Part model, mm, in its own coordinate system. A direction names the side the tool comes from. Give positions to 0.01 mm unless a question says otherwise; leave off trailing zeros. Order: outer loops, then holes, each group sorted by start corner. A loop starts at its lowest first (then second) coordinate and runs counter-clockwise, first axis right, second up. Notation, with made-up numbers: M -29.75,56.5 L 4.25,56.5 A22 cw 4.25,74.5 Z; hole C -37,56 d7. An arc over 180 degrees is marked long. Answer as a JSON object with one key per item and string values.
from build123d import *

# Parameters (mm, degrees)
BOSS_EXTRUDE1_DEPTH = 20
CUT_EXTRUDE3_DEPTH  = 8
SKETCH4_W           = 7
SKETCH4_H           = 15
SKETCH4_R           = 2
BOSS_EXTRUDE2_DEPTH = 5


with BuildPart() as part:
    # Sketch1 → Boss-Extrude1 (new body)
    with BuildSketch(Plane(origin=(0, 0, 0), x_dir=(1, 0, 0), z_dir=(0, 1, 0))):
        Polygon((-1.5, -12.5), (-1.5, 4.5), (1.5, 4.5), (1.5, -12.5), (3.5, -12.5), (3.5, 12.5), (-3.5, 12.5), (-3.5, -12.5), align=None)
    extrude(amount=BOSS_EXTRUDE1_DEPTH)

    # Sketch2 → Cut-Extrude3 (cut)
    with BuildSketch(Plane.XY.offset(-4.5)):
        with BuildLine():
            Line((2, 17.5), (2, 10.5))
            ThreePointArc((2, 10.5), (0, 8.5), (-2, 10.5))
            Line((-2, 10.5), (-2, 17.5))
            ThreePointArc((-2, 17.5), (0, 19.5), (2, 17.5))
        make_face()
    extrude(amount=-CUT_EXTRUDE3_DEPTH, mode=Mode.SUBTRACT)

    # Sketch4 → Boss-Extrude2 (add)
    with BuildSketch(Plane(origin=(0, 0, -12.5), x_dir=(-1, 0, 0), z_dir=(0, 0, -1))):
        with Locations((0, -7.5)):
            Rectangle(SKETCH4_W, SKETCH4_H)
        with Locations((0, -4)):
            Circle(SKETCH4_R, mode=Mode.SUBTRACT)
        with Locations((0, -11)):
            Circle(SKETCH4_R, mode=Mode.SUBTRACT)
    extrude(amount=-BOSS_EXTRUDE2_DEPTH)


solid = part.part
1. Cut at A-A on y = -4. Give the cut face in (x, z).
Worked answers:
{"outline": "M -3.5,-12.5 L -2,-12.5 L -2,-7.5 L -3.5,-7.5 Z; M 2,-12.5 L 3.5,-12.5 L 3.5,-7.5 L 2,-7.5 Z"}
2. Cut at D-D on x = 0.5. Give the cut face in (y, z), plus the area to 3 significant figures.
Worked answers:
{"outline": "M -15,-12.5 L -12.94,-12.5 L -12.94,-7.5 L -15,-7.5 Z; M -9.06,-12.5 L -5.94,-12.5 L -5.94,-7.5 L -9.06,-7.5 Z; M -2.06,-12.5 L 8.56,-12.5 L 8.56,-4.5 L 0,-4.5 L 0,-7.5 L -2.06,-7.5 Z; M 19.44,-12.5 L 20,-12.5 L 20,-4.5 L 19.44,-4.5 Z", "area": "109 mm^2"}
3. Cut at B-B on z = -2.25. Give the cut face in (x, y), plus the area to 3 significant figures.
Worked answers:
{"outline": "M -3.5,0 L -1.5,0 L -1.5,20 L -3.5,20 Z; M 1.5,0 L 3.5,0 L 3.5,20 L 1.5,20 Z", "area": "80.0 mm^2"}
4. Cut at C-C on y = 2.5. Give the cut face in (x, z).
Worked answers:
{"outline": "M -3.5,-12.5 L 3.5,-12.5 L 3.5,12.5 L 1.5,12.5 L 1.5,-4.5 L -1.5,-4.5 L -1.5,12.5 L -3.5,12.5 Z"}
5. Pin check, flat tips, straight feed: P1, Ø4, axis at x = -2.5, z = 9.5, coming from the -Y side; P2, Ø3.5, axis at x = -0.5, y = -4.5, coming from the +Z side. Stop position of each tip, or through.
Worked answers:
{"P1": "stops at y = 0", "P2": "stops at z = -7.5"}
6. Two-plate mould, pull along X, no slides. Class faces 6 (the cylindrical face through (0, 19.5, -8.4)), 7 (the flat face through (2, 20, 0)), 8 (the flat face through (3.5, 6, -3)): +X half, -X half, draft (parallel to the pull), parting line (faces both ways), or undercut.
Worked answers:
{"face 6": "undercut", "face 7": "draft", "face 8": "+X half"}
7. Which spindle directions (+Z, -Z, +X, -X, +Y, -Y) get a long thin tool onto all of the face, cutting with end or side? Do faces 1 (the flat face through (0, -7, -7.5)), 2 (the flat face through (0, 19.7, -4.5)), 3 (the cylindrical face through (0, 8.5, -8.4)), 4 (the flat face through (0, 3, -12.5)), 5 (the flat face through (-3.5, 6, -3)). Say none if no direction does.
Worked answers:
{"face 1": "+Z, +X, -X, -Y", "face 2": "+Z, +Y, -Y", "face 3": "-Z", "face 4": "-Z, +X, -X, +Y, -Y", "face 5": "+Z, -Z, -X, +Y, -Y"}
8. Probe line 1 along Y through (x, z) = (0, -8.6); line 2 along Y through (x, z) = (0.75, -11); line 3 along X through (y, z) = (7, 9.75). List the from-to ranges inside material, lowest first.
Worked answers:
{"line 1": "y = -15 to -13, -9 to -6, -2 to 8.5, 19.5 to 20", "line 2": "y = -15 to -12.85, -9.15 to -5.85, -2.15 to 8.65, 19.35 to 20", "line 3": "x = -3.5 to -1.5, 1.5 to 3.5"}
